```python
from build123d import *

# Parameters (mm, degrees)
SKETCH1_R           = 9.525
BOSS_EXTRUDE1_DEPTH = 63.5
SKETCH2_OUTSIDE_W   = 34.846
SKETCH2_OUTSIDE_H   = 34.846
CUT_EXTRUDE1_DEPTH  = 31.75
SKETCH3_R           = 11.1125
BOSS_EXTRUDE2_DEPTH = 63.5
SKETCH4_R           = 9.525
BOSS_EXTRUDE3_DEPTH = 16.637
CUT_EXTRUDE2_DEPTH  = 63.5


with BuildPart() as part:
    # Sketch1 → Boss-Extrude1 (new body)
    with BuildSketch(Plane(origin=(0, 0, 0), x_dir=(0, 0, -1), z_dir=(1, 0, 0))):
        Circle(SKETCH1_R)
    extrude(amount=BOSS_EXTRUDE1_DEPTH)

    # Sketch2 outside → Cut-Extrude1 (cut)
    with BuildSketch(Plane(origin=(63.5, 0, 0), x_dir=(0, 0, -1), z_dir=(1, 0, 0))):
        Rectangle(SKETCH2_OUTSIDE_W, SKETCH2_OUTSIDE_H)
        with BuildLine():
            Line((-2.10185, -8.219105519), (-2.10185, -9.277180491))
            ThreePointArc((-2.10185, -9.277180491), (-1.488051562, -9.395187802), (-0.867828293, -9.472630329))
            Line((-0.867828293, -9.472630329), (-0.540865145, -8.466341232))
            ThreePointArc((-0.540865145, -8.466341232), (0, -8.4836), (0.540865145, -8.466341232))
            Line((0.540865145, -8.466341232), (0.867828293, -9.472630329))
            ThreePointArc((0.867828293, -9.472630329), (1.488051562, -9.395187802), (2.10185, -9.277180491))
            Line((2.10185, -9.277180491), (2.10185, -8.219105519))
            ThreePointArc((2.10185, -8.219105519), (2.621576573, -8.068383062), (3.130636642, -7.884832476))
            Line((3.130636642, -7.884832476), (3.752557506, -8.74083311))
            ThreePointArc((3.752557506, -8.74083311), (4.318493831, -8.47552136), (4.86578457, -8.173615589))
            Line((4.86578457, -8.173615589), (4.538821423, -7.167326493))
            ThreePointArc((4.538821423, -7.167326493), (4.986534966, -6.863376573), (5.413959611, -6.531501381))
            Line((5.413959611, -6.531501381), (6.269960245, -7.153422245))
            ThreePointArc((6.269960245, -7.153422245), (6.726211835, -6.726211835), (7.153422245, -6.269960245))
            Line((7.153422245, -6.269960245), (6.531501381, -5.413959611))
            ThreePointArc((6.531501381, -5.413959611), (6.863376573, -4.986534966), (7.167326493, -4.538821423))
            Line((7.167326493, -4.538821423), (8.173615589, -4.86578457))
            ThreePointArc((8.173615589, -4.86578457), (8.47552136, -4.318493831), (8.74083311, -3.752557506))
            Line((8.74083311, -3.752557506), (7.884832476, -3.130636642))
            ThreePointArc((7.884832476, -3.130636642), (8.068383062, -2.621576573), (8.219105519, -2.10185))
            Line((8.219105519, -2.10185), (9.277180491, -2.10185))
            ThreePointArc((9.277180491, -2.10185), (9.395187802, -1.488051562), (9.472630329, -0.867828293))
            Line((9.472630329, -0.867828293), (8.466341232, -0.540865145))
            ThreePointArc((8.466341232, -0.540865145), (8.4836, 0), (8.466341232, 0.540865145))
            Line((8.466341232, 0.540865145), (9.472630329, 0.867828293))
            ThreePointArc((9.472630329, 0.867828293), (9.395187802, 1.488051562), (9.277180491, 2.10185))
            Line((9.277180491, 2.10185), (8.219105519, 2.10185))
            ThreePointArc((8.219105519, 2.10185), (8.068383062, 2.621576573), (7.884832476, 3.130636642))
            Line((7.884832476, 3.130636642), (8.74083311, 3.752557506))
            ThreePointArc((8.74083311, 3.752557506), (8.47552136, 4.318493831), (8.173615589, 4.86578457))
            Line((8.173615589, 4.86578457), (7.167326493, 4.538821423))
            ThreePointArc((7.167326493, 4.538821423), (6.863376573, 4.986534966), (6.531501381, 5.413959611))
            Line((6.531501381, 5.413959611), (7.153422245, 6.269960245))
            ThreePointArc((7.153422245, 6.269960245), (6.726211835, 6.726211835), (6.269960245, 7.153422245))
            Line((6.269960245, 7.153422245), (5.413959611, 6.531501381))
            ThreePointArc((5.413959611, 6.531501381), (4.986534966, 6.863376573), (4.538821423, 7.167326493))
            Line((4.538821423, 7.167326493), (4.86578457, 8.173615589))
            ThreePointArc((4.86578457, 8.173615589), (4.318493831, 8.47552136), (3.752557506, 8.74083311))
            Line((3.752557506, 8.74083311), (3.130636642, 7.884832476))
            ThreePointArc((3.130636642, 7.884832476), (2.621576573, 8.068383062), (2.10185, 8.219105519))
            Line((2.10185, 8.219105519), (2.10185, 9.277180491))
            ThreePointArc((2.10185, 9.277180491), (1.488051562, 9.395187802), (0.867828293, 9.472630329))
            Line((0.867828293, 9.472630329), (0.540865145, 8.466341232))
            ThreePointArc((0.540865145, 8.466341232), (0, 8.4836), (-0.540865145, 8.466341232))
            Line((-0.540865145, 8.466341232), (-0.867828293, 9.472630329))
            ThreePointArc((-0.867828293, 9.472630329), (-1.488051562, 9.395187802), (-2.10185, 9.277180491))
            Line((-2.10185, 9.277180491), (-2.10185, 8.219105519))
            ThreePointArc((-2.10185, 8.219105519), (-2.621576573, 8.068383062), (-3.130636642, 7.884832476))
            Line((-3.130636642, 7.884832476), (-3.752557506, 8.74083311))
            ThreePointArc((-3.752557506, 8.74083311), (-4.318493831, 8.47552136), (-4.86578457, 8.173615589))
            Line((-4.86578457, 8.173615589), (-4.538821423, 7.167326493))
            ThreePointArc((-4.538821423, 7.167326493), (-4.986534966, 6.863376573), (-5.413959611, 6.531501381))
            Line((-5.413959611, 6.531501381), (-6.269960245, 7.153422245))
            ThreePointArc((-6.269960245, 7.153422245), (-6.726211835, 6.726211835), (-7.153422245, 6.269960245))
            Line((-7.153422245, 6.269960245), (-6.531501381, 5.413959611))
            ThreePointArc((-6.531501381, 5.413959611), (-6.863376573, 4.986534966), (-7.167326493, 4.538821423))
            Line((-7.167326493, 4.538821423), (-8.173615589, 4.86578457))
            ThreePointArc((-8.173615589, 4.86578457), (-8.47552136, 4.318493831), (-8.74083311, 3.752557506))
            Line((-8.74083311, 3.752557506), (-7.884832476, 3.130636642))
            ThreePointArc((-7.884832476, 3.130636642), (-8.068383062, 2.621576573), (-8.219105519, 2.10185))
            Line((-8.219105519, 2.10185), (-9.277180491, 2.10185))
            ThreePointArc((-9.277180491, 2.10185), (-9.395187802, 1.488051562), (-9.472630329, 0.867828293))
            Line((-9.472630329, 0.867828293), (-8.466341232, 0.540865145))
            ThreePointArc((-8.466341232, 0.540865145), (-8.4836, 0), (-8.466341232, -0.540865145))
            Line((-8.466341232, -0.540865145), (-9.472630329, -0.867828293))
            ThreePointArc((-9.472630329, -0.867828293), (-9.395187802, -1.488051562), (-9.277180491, -2.10185))
            Line((-9.277180491, -2.10185), (-8.219105519, -2.10185))
            ThreePointArc((-8.219105519, -2.10185), (-8.068383062, -2.621576573), (-7.884832476, -3.130636642))
            Line((-7.884832476, -3.130636642), (-8.74083311, -3.752557506))
            ThreePointArc((-8.74083311, -3.752557506), (-8.47552136, -4.318493831), (-8.173615589, -4.86578457))
            Line((-8.173615589, -4.86578457), (-7.167326493, -4.538821423))
            ThreePointArc((-7.167326493, -4.538821423), (-6.863376573, -4.986534966), (-6.531501381, -5.413959611))
            Line((-6.531501381, -5.413959611), (-7.153422245, -6.269960245))
            ThreePointArc((-7.153422245, -6.269960245), (-6.726211835, -6.726211835), (-6.269960245, -7.153422245))
            Line((-6.269960245, -7.153422245), (-5.413959611, -6.531501381))
            ThreePointArc((-5.413959611, -6.531501381), (-4.986534966, -6.863376573), (-4.538821423, -7.167326493))
            Line((-4.538821423, -7.167326493), (-4.86578457, -8.173615589))
            ThreePointArc((-4.86578457, -8.173615589), (-4.318493831, -8.47552136), (-3.752557506, -8.74083311))
            Line((-3.752557506, -8.74083311), (-3.130636642, -7.884832476))
            ThreePointArc((-3.130636642, -7.884832476), (-2.621576573, -8.068383062), (-2.10185, -8.219105519))
        make_face(mode=Mode.SUBTRACT)
    extrude(amount=-CUT_EXTRUDE1_DEPTH, mode=Mode.SUBTRACT)

    # Sketch3 → Boss-Extrude2 (add)
    with BuildSketch(Plane.ZY):
        Circle(SKETCH3_R)
    extrude(amount=BOSS_EXTRUDE2_DEPTH)

    # Sketch4 → Boss-Extrude3 (add)
    with BuildSketch(Plane.ZY.offset(63.5)):
        Circle(SKETCH4_R)
    extrude(amount=BOSS_EXTRUDE3_DEPTH)

    # Sketch5 → Cut-Extrude2 (cut)
    with BuildSketch(Plane.ZY.offset(63.5)):
        with BuildLine():
            Line((0, 8.7249), (2.3876, 8.7249))
            Line((2.3876, 8.7249), (2.3876, 10.852972979))
            ThreePointArc((2.3876, 10.852972979), (0, 11.1125), (-2.3876, 10.852972979))
            Line((-2.3876, 10.852972979), (-2.3876, 8.7249))
            Line((-2.3876, 8.7249), (0, 8.7249))
        make_face()
    extrude(amount=-CUT_EXTRUDE2_DEPTH, mode=Mode.SUBTRACT)


solid = part.part
```
Can you work these out from the model? Positions are in its coordinate system, mm. A direction names the side the tool comes from. Round coordinates to 2 decimals unless told otherwise and drop trailing zeros. Loops run counter-clockwise (first coordinate to the right, second up) from the corner with the lowest first, then second, coordinate; pieces in that order, holes last. Notation, with made-up numbers: M 79,66.25 L 83,66.25 A33 cw 83,105.25 Z; hole C 34.5,87 d1. An arc over 180 degrees is marked long. Write item = value, one per line. Start each with the question number.
(1) If we mould it in two halves opening along Z, with no side actions, what happens to faces 4 (the face through (-71.702, -5.796, -7.559)), 5 (the face through (31.75, 7.1, 5)), 6 (the face through (-32, 8.725, 0)), 7 (the face through (63.5, 0, 0))? For each: released by +Z, released by -Z, zero draft, split by the parting line, or undercut.
(2) Suppose I cut it at A-A on x = -9.5. Write out the boundary of the cut face in (y, z) (1 decimal), plus the area to 3 significant figures.
(3) Which directions (+Z, -Z, +X, -X, +Y, -Y) give clear straight access to the entire face, cutting with the end or side of a thin tool? Please do faces 1 (the face through (15.653, -5.796, 7.559)), 2 (the face through (-63.5, -5, -8.3)), 3 (the face through (-80.137, 0, 0)).
(4) I need wall thicknesses on line 1 along Y through (x, z) = (-60.5, 10); line 2 along Z through (x, y) = (15, 1); line 3 along Y through (x, z) = (46, -3.75). Which ranges of each line are inside material? Lowest first, please.
(5) I'm going to push flat-ended pins straight in: P1, Ø0.8, axis at x = 45, z = -9, coming from the -Y side; P2, Ø1.5, axis at x = -54, y = 5, coming from the -Z side; P3, Ø1.2, axis at x = 51, y = -8.5, coming from the +Z side; P4, Ø3, axis at x = -30.5, y = 1.5, coming from the +Z side. Where does each tip first touch, or does it pass through?
Answer block:
q1.face_4 = split by the parting line
q1.face_5 = undercut
q1.face_6 = undercut
q1.face_7 = zero draft
q2.outline = M 8.7,-2.4 L 8.7,2.4 L 10.9,2.4 A11.1 ccw long 10.9,-2.4 Z
q2.area = 377 mm²
q3.face_1 = +X
q3.face_2 = -X
q3.face_3 = +Z, -Z, -X, +Y, -Y
q4.line_1 = -4.85 to 4.85
q4.line_2 = -9.47 to 9.47
q4.line_3 = -8.74 to 8.74
q5.P1 = -4.06
q5.P2 = -10.27
q5.P3 = 4.87
q5.P4 = 11.11
